Part model, mm, in its own coordinate system. Face numbers are marked on the shaded views. A direction names the side the tool comes from. Coordinates: 2 decimals unless noted, no trailing zeros. Loops run counter-clockwise (first coordinate to the right, second up) from the corner with the lowest first, then second, coordinate; pieces in that order, holes last. Notation, with made-up numbers: (22.25, 89.25) -> (47.25, 89.25) arc R24 cw to (47.25, 111.25) -> close; hole circle Ø8 at (-36.5, 7.25). An arc over 180 degrees is marked (long way). One line per question, with ' | ' between items. Start each with the question number.
1) 3-axis set-ups, long thin cutter, end or side, ignore diameter. For the marked faces 1 and 2: which of +Z, -Z, +X, -X, +Y, -Y reach the whole face in a straight line?
2) Cut at A-A (z = 17.5). List the corners of the cut face in (x, y).
3) Probe L1, parallel to Z at x = -7, y = -28.5; L2, parallel to Y at x = 33.5, z = 9.5; L3, parallel to Y at x = -3.5, z = 18.5. List the from-to ranges inside material, lowest first. Write a range as from..to.
4) Drop flat-ended pins along their axis: pin 1 (12 mm diameter, centred on x = 3, z = 0.5, fed in from -Y); pin 2 (12 mm diameter, centred on x = 37, z = 13.5, fed in from -Y) (3 decimals); pin 3 (1.5 mm diameter, centred on y = 5.5, z = 5.5, fed in from +X). Give the stop position or say it passes through.
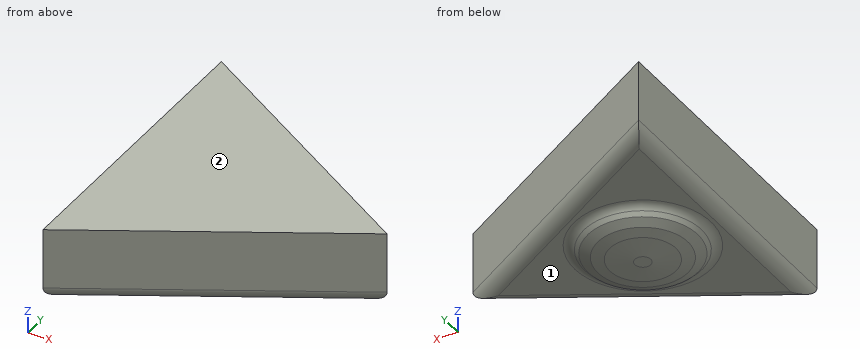
from build123d import *

# Parameters (mm, degrees)
F1_DEPTH    = 29.464
F2_R        = 23.506947033
F3_DEPTH    = 36.322
F4_SIZE     = 5.08
F5_T3_DEPTH = 143.4285494589
F5_T5_DEPTH = 137.562670724
F5_T7_DEPTH = 131.696791989
F6_SIZE     = 5.08
F7_SIZE     = 5.08
F8_SIZE     = 5.08


# Not quite as in the source:
# - a fillet or chamfer that OpenCascade refuses, or shapes differently, is made with other operations: its cross-section is extruded or revolved along the edge and cut away or added


with BuildPart() as f1:
    # F0 (on Top) → F1 (new body)
    with BuildSketch(Plane.XY):
        Polygon((-34.0719074011, 59.0142747295), (-34.0719074011, -59.0142747295), (68.1438148022, 0), align=None)
    extrude(amount=F1_DEPTH)

    # F2 (on face) → F3 (join)
    with BuildSketch(Plane.XY.offset(29.464)):
        Circle(F2_R)
    extrude(amount=-F3_DEPTH)

    # F4
    f4_edges = [f1.edges().sort_by_distance(p)[0] for p in [
        (-23.506947, 0, -6.858),
    ]]
    chamfer(f4_edges, length=F4_SIZE)

    # F5: fillet of radius 5.08 on 4 edges, made by hand

    # F5_s1 → F5_t2 (revolve)
    with BuildSketch(Plane.XZ):
        with BuildLine():
            ThreePointArc((23.506947033, -1.778), (25.2422963406, -0.4658608604), (27.367412808, 0))
            Line((27.367412808, 0), (23.506947033, 0))
            Line((23.506947033, 0), (23.506947033, -1.778))
        make_face()
    revolve(axis=Axis((0, 0, 0), (0, 0, 1)))

    # F5_s4 → F5_t3 (cut)
    with BuildSketch(Plane(origin=(62.1063837297, -35.8571373647, 0), x_dir=(0, 0, 1), z_dir=(-0.8660254038, 0.5, 0))):
        with BuildLine():
            ThreePointArc((0, 28.9919074011), (1.4878975516, 32.5840098495), (5.08, 34.0719074011))
            Line((5.08, 34.0719074011), (0, 34.0719074011))
            Line((0, 34.0719074011), (0, 28.9919074011))
        make_face()
    extrude(amount=F5_T3_DEPTH, mode=Mode.SUBTRACT)

    # F5_s6 → F5_t5 (cut)
    with BuildSketch(Plane(origin=(-62.1063837297, -35.8571373647, 0), x_dir=(0, 0, 1), z_dir=(0.8660254038, 0.5, 0))):
        with BuildLine():
            ThreePointArc((0, 28.9919074011), (1.4878975516, 32.5840098495), (5.08, 34.0719074011))
            Line((5.08, 34.0719074011), (0, 34.0719074011))
            Line((0, 34.0719074011), (0, 28.9919074011))
        make_face()
    extrude(amount=F5_T5_DEPTH, mode=Mode.SUBTRACT)

    # F5_s8 → F5_t7 (cut)
    with BuildSketch(Plane.XZ.offset(-65.8483959945)):
        with BuildLine():
            ThreePointArc((-28.9919074011, 0), (-32.5840098495, 1.4878975516), (-34.0719074011, 5.08))
            Line((-34.0719074011, 5.08), (-34.0719074011, 0))
            Line((-34.0719074011, 0), (-28.9919074011, 0))
        make_face()
    extrude(amount=F5_T7_DEPTH, mode=Mode.SUBTRACT)

    # F6
    f6_edges = [f1.edges().sort_by_distance(p)[0] for p in [
        (-18.426947, 0, -6.858),
    ]]
    chamfer(f6_edges, length=F6_SIZE)

    # F7
    f7_edges = [f1.edges().sort_by_distance(p)[0] for p in [
        (-13.346947, 0, -6.858),
    ]]
    chamfer(f7_edges, length=F7_SIZE)

    # F8
    f8_edges = [f1.edges().sort_by_distance(p)[0] for p in [
        (-8.266947, 0, -6.858),
    ]]
    chamfer(f8_edges, length=F8_SIZE)


solid = f1.part
Reported:
1) face 1: -Z | face 2: +Z, +X, -X, +Y, -Y
2) outline: (-34.07, -59.01) -> (68.14, 0) -> (-34.07, 59.01) -> close
3) L1: z = 0..29.46 | L2: y = -20..20 | L3: y = -41.36..41.36
4) pin 1: stops at y = -40.32 | pin 2: stops at y = -21.445 | pin 3: stops at x = 59.92
